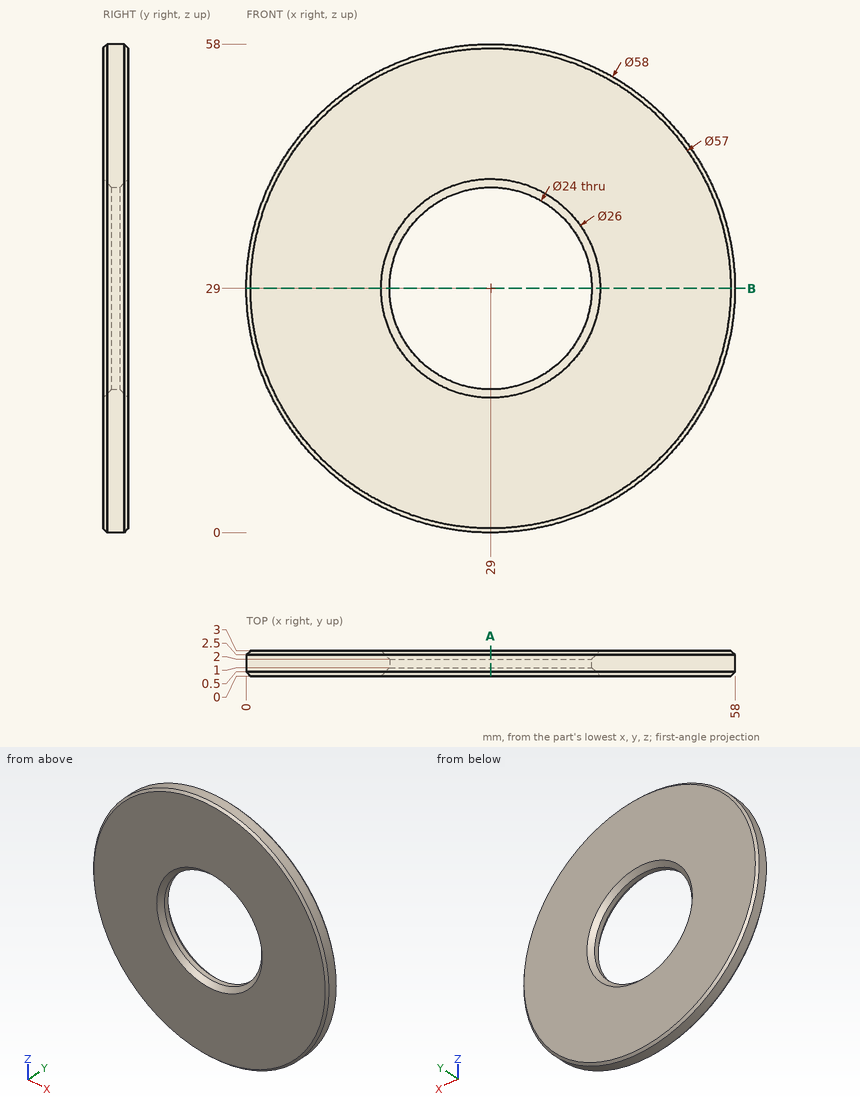
Answer from the drawing. Dimensions are ordinates in mm from the lowest x, y and z of the part. Give positions to 0.01 mm unless a question says otherwise; leave off trailing zeros. Write each loop counter-clockwise with the first axis right and the second up, starting at its lowest first coordinate (ties: lowest second). Pieces come first, ordered by that corner, then holes. Notation, with made-up numbers: (0.5, 71.25) - (35.5, 71.25) arc R15 cw to (35.5, 96.25) - close; hole circle Ø2 at (75, 3.25). An arc over 180 degrees is marked (long way). Answer in a Markdown table with one row per item. Add a question column.
Item 1: Section B-B, the plane z = 29 is taken. Write down the section's boundary in (x, y), and give its area (3 significant figures).
Item 2: Find the intervals of material crossed by L1, parallel to Z at x = 29, y = 1.2; L2, parallel to Z at x = 29.5, y = 0.8; L3, parallel to X at y = 2.75, z = 7.5, in increasing order.
Item 3: Flat-ended cylindrical pins translate along their axes: P1, Ø1, axis at x = 25, z = 17.5, coming from the +Y side; P2, Ø19, axis at x = 29, z = 29, coming from the -Y side; P3, Ø2, axis at x = 24, z = 39.5, coming from the +Y side. Find the tip coordinate at first contact, or state that the pin passes through.
Item 4: Section A-A, the plane x = 29 is taken. Write down the section's boundary in (y, z).
Recorded:
| question | item | result |
|---|---|---|
| 1 | outline | (0, 0.5) - (0.5, 0) - (16, 0) - (17, 1) - (17, 2) - (16, 3) - (0.5, 3) - (0, 2.5) - close; (41, 1) - (42, 0) - (57.5, 0) - (58, 0.5) - (58, 2.5) - (57.5, 3) - (42, 3) - (41, 2) - close |
| 1 | area | 99.5 mm2 |
| 2 | L1 | z = 0 to 17, 41 to 58 |
| 2 | L2 | z = 0 to 16.81, 41.19 to 58 |
| 2 | L3 | x = 9.91 to 48.09 |
| 3 | P1 | stops at y = 2.68 |
| 3 | P2 | passes through |
| 3 | P3 | stops at y = 2.63 |
| 4 | outline | (0, 0.5) - (0.5, 0) - (2.5, 0) - (3, 0.5) - (3, 16) - (2, 17) - (1, 17) - (0, 16) - close; (0, 42) - (1, 41) - (2, 41) - (3, 42) - (3, 57.5) - (2.5, 58) - (0.5, 58) - (0, 57.5) - close |
